The listing builds one solid part. Answer for the finished solid, in the listing's coordinates (mm). Give positions to 0.01 mm unless a question says otherwise; leave off trailing zeros. Write each loop counter-clockwise with the first axis right and the second up, starting at its lowest first coordinate (ties: lowest second). Pieces come first, ordered by that corner, then holes. Notation, with made-up numbers: (6.5, 37.5) - (21.5, 37.5) arc R11 cw to (21.5, 44.5) - close; hole circle Ø7 at (-13.75, 78). An arc over 180 degrees is marked (long way). One line per item, written item: value. Start each with the question number.
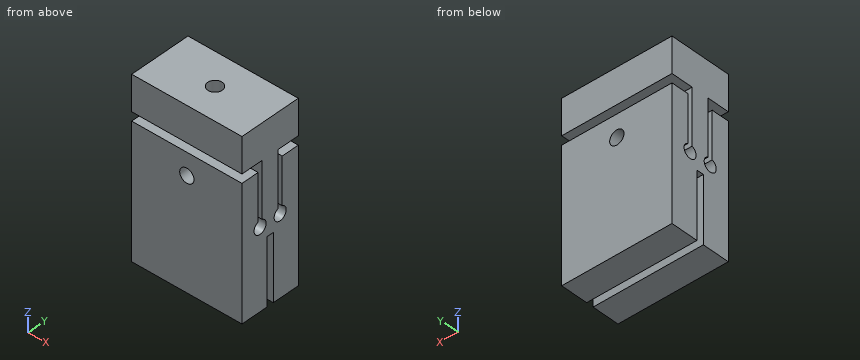
Autodesk Inventor part; units mm, degrees
ref_plane "YZ Plane" through (0, 0, 0) normal (1, 0, 0) x (0, 1, 0)
ref_plane "XZ Plane" through (0, 0, 0) normal (0, 1, 0) x (-1, 0, 0)
ref_plane "XY Plane" through (0, 0, 0) normal (0, 0, 1) x (1, 0, 0)
sketch "Sketch1" plane through (0, 0, 0) normal (0, 0, 1) x (1, 0, 0)
  line L0 (12.5, -7) -> (-12.5, -7)
  line L1 (-12.5, -7) -> (-12.5, 7)
  line L2 (-12.5, 7) -> (12.5, 7)
  line L3 (12.5, 7) -> (12.5, -7)
  line L4 (12.5, -7) -> (-12.5, 7) construction
  line L5 (-12.5, -7) -> (12.5, 7) construction
  point P0 (0, 0)
  dimension "d0" = 25
  dimension "d1" = 14
extrude "Extrusion1" add sketch "Sketch1" along normal blind 30
sketch "Sketch2" plane through (0, 0, 0) normal (0, 0, -1) x (-1, 0, 0)
  line L0 (15, -0.8) -> (-15, -0.8)
  line L1 (-15, -0.8) -> (-15, 0.8)
  line L2 (-15, 0.8) -> (15, 0.8)
  line L3 (15, 0.8) -> (15, -0.8)
  line L4 (15, -0.8) -> (-15, 0.8) construction
  line L5 (-15, -0.8) -> (15, 0.8) construction
  point P0 (0, 0)
  dimension "d4" = 30
  dimension "d5" = 1.6
extrude "Extrusion2" cut sketch "Sketch2" against normal blind 15
sketch "Sketch4" plane through (12.5, -7, 30) normal (1, 0, 0) x (0, 0, -1)
  line L0 (-12, 4.5) -> (12, 4.5)
  line L1 (12, 4.5) -> (12, 9.5)
  line L2 (12, 9.5) -> (-12, 9.5)
  line L3 (-12, 9.5) -> (-12, 4.5)
  line L4 (0, 0) -> (0, 14)
  line L5 (-12, 4.5) -> (12, 9.5) construction
  line L6 (12, 4.5) -> (-12, 9.5) construction
  line L7 (30, 0) -> (0, 0)
  circle A0 centre (12, 9.5) radius 1.5
  circle A1 centre (12, 4.5) radius 1.5
  line L8 (-12, 9) -> (12, 9)
  line L9 (12, 9) -> (12, 10)
  line L10 (12, 10) -> (-12, 10)
  line L11 (-12, 10) -> (-12, 9)
  line L12 (0, 14) -> (0, 0)
  line L13 (-12, 9) -> (12, 10) construction
  line L14 (12, 9) -> (-12, 10) construction
  line L15 (-12, 4) -> (12, 4)
  line L16 (12, 4) -> (12, 5)
  line L17 (12, 5) -> (-12, 5)
  line L18 (-12, 5) -> (-12, 4)
  line L19 (-12, 4) -> (12, 5) construction
  line L20 (12, 4) -> (-12, 5) construction
  point P0 (30, 7)
  point P1 (0, 7)
  point P2 (0, 9.5)
  point P3 (0, 4.5)
  point P4 (10.5858, 5)
  point P5 (10.5858, 4)
  point P6 (10.5858, 10)
  point P7 (-12, 9)
  point P8 (10.5858, 9)
  dimension "d16" = 5
  dimension "d17" = 3
  dimension "d18" = 3
  dimension "d19" = 1
  dimension "d20" = 1
  dimension "d23" = 12
extrude "Extrusion3" cut sketch "Sketch4" against normal through all contours L3 L17 L4 L0 | L0 L4 L15 L18 | L4 L17 A1 L0 | L0 A1 L15 L4 | A1 L17 L1 L0 | L0 L16 L15 A1 | L3 L2 L4 L8 | L1 A1 L15 L16 | A1 L1 L17 | L4 L2 A0 L8 | L11 L10 L4 L2 | L4 L10 A0 L2 | L8 L1 A0 | A0 L2 L1 L8 | L1 L9 L10 A0 | A0 L10 L9 L2
sketch "Sketch5" plane through (-12.5, 7, 0) normal (0, 1, 0) x (1, 0, 0)
  line L0 (25, -30) -> (0, -30)
  point P0 (12.5, 0)
  point P1 (12.5, -25)
  point P2 (12.5, -30)
  dimension "d24" = 5
sketch "Sketch6" plane through (-12.5, -7, 0) normal (0, -1, 0) x (1, 0, 0)
  point P0 (12.5, 0)
  point P1 (12.5, 25)
hole "Hole2" at (0, -7, 25) direction (0, 1, 0) diameter 3.242 depth 4
hole "Hole3" at (0, 7, 25) direction (0, -1, 0) diameter 3.242 depth 4
sketch "Sketch7" plane through (0, 0, 30) normal (0, 0, 1) x (1, 0, 0)
  line L0 (-12.5, -2) -> (12.5, -2)
  line L1 (12.5, -2) -> (12.5, 2)
  line L2 (12.5, 2) -> (-12.5, 2)
  line L3 (-12.5, 2) -> (-12.5, -2)
  point P0 (0, 0)
extrude "Extrusion4" add sketch "Sketch7" along normal blind 2
sketch "Sketch11" plane through (0, 0, 32) normal (0, 0, 1) x (1, 0, 0)
  line L0 (-12.5, 7) -> (-12.5, 0.8)
  line L1 (12.5, -7) -> (-12.5, -7)
  line L2 (-12.5, -7) -> (-12.5, 7)
  line L3 (-12.5, 7) -> (12.5, 7)
  line L4 (12.5, 7) -> (12.5, -7)
  line L5 (12.5, -7) -> (-12.5, 7) construction
  line L6 (-12.5, -7) -> (12.5, 7) construction
  point P0 (0, 0)
  point P1 (-12.5, 0.8)
extrude "Extrusion6" add sketch "Sketch11" along normal blind 8
sketch "Sketch12" plane through (0, 0, 40) normal (0, 0, 1) x (1, 0, 0)
  point P0 (0, 0)
  point P1 (0, 0)
hole "Hole4" at (0, 0, 40) direction (0, 0, -1) diameter 3.242 depth 7
properties part number "holder_slide_1.5mmThick_25mmWide"
Item 1: Straight lines are drawn through the part: line 1 along Z through (x, y) = (0, -4.95); line 2 along Y through (x, z) = (5, 20); line 3 along Z through (x, y) = (5.25, -6). For each, find the intervals that lie inside material, in ascending order.
Item 2: Find section A-A on y = -5.5. Determine the outline of the cut face in (x, z).
Item 3: Find section D-D on z = 25. Determine the outline of the cut face in (x, y), plus the area to 3 significant figures.
Item 4: Find section B-B on z = 8.5. Determine the outline of the cut face in (x, y).
Item 5: This flat-tipped pin is pushed along its axis until it touches: pin 1 Ø1.3 at (x, y) = (-2.5, 0.5) entering from -Z. Where does it stop, or does it pass through?
Item 6: Find section C-C on y = -2.5. Determine the outline of the cut face in (x, z), plus the area to 4 significant figures.
Values:
1. line 1: 0 to 23.38, 26.62 to 30, 32 to 40
1. line 2: -7 to -3, -2 to 2, 3 to 7
1. line 3: 0 to 30, 32 to 40
2. outline: (-12.5, 0) - (12.5, 0) - (12.5, 30) - (-12.5, 30) - close; (-12.5, 32) - (12.5, 32) - (12.5, 40) - (-12.5, 40) - close; hole circle Ø3.24 at (0, 25)
3. outline: (-12.5, -7) - (-1.62, -7) - (-1.62, -3) - (-12.5, -3) - close; (-12.5, -2) - (12.5, -2) - (12.5, 2) - (-12.5, 2) - close; (-12.5, 3) - (-1.62, 3) - (-1.62, 7) - (-12.5, 7) - close; (1.62, -7) - (12.5, -7) - (12.5, -3) - (1.62, -3) - close; (1.62, 3) - (12.5, 3) - (12.5, 7) - (1.62, 7) - close
3. area: 274 mm^2
4. outline: (-12.5, -7) - (12.5, -7) - (12.5, -0.8) - (-12.5, -0.8) - close; (-12.5, 0.8) - (12.5, 0.8) - (12.5, 7) - (-12.5, 7) - close
5. pin 1: z = 0
6. outline: (-12.5, 0) - (12.5, 0) - (12.5, 16.5) - (-12.5, 16.5) - close; (-12.5, 32) - (12.5, 32) - (12.5, 40) - (-12.5, 40) - close
6. area: 612.5 mm^2
